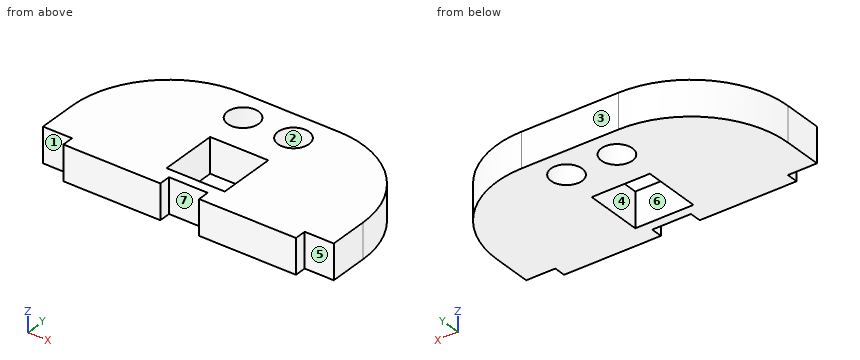
```python
from build123d import *

# Parameters (mm, degrees)
ESQUISSE1_R        = 8
ESQUISSE1_W        = 30
ESQUISSE1_H        = 30
BOSS_EXTRU_1_DEPTH = 18


with BuildPart() as part:
    # Esquisse1 → Boss.-Extru.1 (new body)
    with BuildSketch(Plane.XY):
        with BuildLine():
            Line((0, 0), (0, 20))
            ThreePointArc((0, 20), (14.644660941, 55.355339059), (50, 70))
            Line((50, 70), (100, 70))
            ThreePointArc((100, 70), (135.355339059, 55.355339059), (150, 20))
            Line((150, 20), (150, 0))
            Line((150, 0), (135, 0))
            Line((135, 0), (135, -6))
            Line((135, -6), (85, -6))
            Line((85, -6), (85, 0))
            Line((85, 0), (65, 0))
            Line((65, 0), (65, -6))
            Line((65, -6), (15, -6))
            Line((15, -6), (15, 0))
            Line((15, 0), (0, 0))
        make_face()
        with Locations((62, 55)):
            Circle(ESQUISSE1_R, mode=Mode.SUBTRACT)
        with Locations((88, 55)):
            Circle(ESQUISSE1_R, mode=Mode.SUBTRACT)
        with Locations((75, 20)):
            Rectangle(ESQUISSE1_W, ESQUISSE1_H, mode=Mode.SUBTRACT)
    extrude(amount=BOSS_EXTRU_1_DEPTH)


solid = part.part
```
The listing builds one solid part. Answer for the finished solid, in the listing's coordinates (mm). Face numbers are marked on the shaded views. A direction names the side the tool comes from. Coordinates: 2 decimals unless noted, no trailing zeros. Write each loop counter-clockwise with the first axis right and the second up, starting at its lowest first coordinate (ties: lowest second). Pieces come first, ordered by that corner, then holes.
Q1. The mould has two halves that part along Y. Classify the marked faces 1, 2, 3 and 4: released by +Y, released by -Y, zero draft, split by the parting line, or undercut.
Returned:
face 1: released by -Y
face 2: undercut
face 3: released by +Y
face 4: undercut
Q2. Find the intervals of material crossed by line 1 along Y through (x, z) = (62, 7.5); line 2 along X through (y, z) = (49, 3); line 3 along X through (y, z) = (14, 11.25), in increasing order.
Returned:
line 1: y = -6 to 5, 35 to 47, 63 to 70
line 2: x = 9.27 to 56.71, 67.29 to 82.71, 93.29 to 140.73
line 3: x = 0 to 60, 90 to 150
Q3. Section D-D, the plane x = 130.5 is taken. Write down the section's boundary in (y, z), then the cut area to 3 significant figures.
Returned:
outline: (-6, 0) - (59.62, 0) - (59.62, 18) - (-6, 18) - close
area: 1,180 mm2
Q4. Section A-A, the plane x = 73.5 is taken. Write down the section's boundary in (y, z).
Returned:
outline: (0, 0) - (5, 0) - (5, 18) - (0, 18) - close; (35, 0) - (70, 0) - (70, 18) - (35, 18) - close
Q5. Which of the six approach directions +Z, -Z, +X, -X, +Y, -Y give full straight-line access (tool end or side, diameter ignored) to the marked faces 5, 6 and 7?
Returned:
face 5: +Z, -Z, +X, -Y
face 6: +Z, -Z
face 7: +Z, -Z, -Y
Q6. Given P1, Ø8, axis at x = 20, y = 43.5, coming from the -Z side; P2, Ø1.8, axis at y = -3.5, z = 12.5, coming from the -X side; P3, Ø2, axis at y = 36, z = 6.5, coming from the +X side; P4, Ø4.5, axis at x = 9.5, z = 6, coming from the -Y side, each flat-ended and moving along its own axis, determine where each tip first touches the part or whether it passes through.
Returned:
P1: stops at z = 0
P2: stops at x = 15
P3: stops at x = 147.7
P4: stops at y = 0
Q7. Section C-C, the plane y = 55 is taken. Write down the section's boundary in (x, z), then the cut area to 3 significant figures.
Returned:
outline: (14.29, 0) - (54, 0) - (54, 18) - (14.29, 18) - close; (70, 0) - (80, 0) - (80, 18) - (70, 18) - close; (96, 0) - (135.71, 0) - (135.71, 18) - (96, 18) - close
area: 1,610 mm2
Q8. Section B-B, the plane z = 11 is taken. Write down the section's boundary in (x, y), then the cut area to 3 significant figures.
Returned:
outline: (0, 0) - (15, 0) - (15, -6) - (65, -6) - (65, 0) - (85, 0) - (85, -6) - (135, -6) - (135, 0) - (150, 0) - (150, 20) arc R50 ccw to (100, 70) - (50, 70) arc R50 ccw to (0, 20) - close; hole circle Ø16 at (62, 55); hole (60, 5) - (90, 5) - (90, 35) - (60, 35) - close; hole circle Ø16 at (88, 55)
area: 8,720 mm2
